Part model, mm, in its own coordinate system. A direction names the side the tool comes from. Coordinates: 2 decimals unless noted, no trailing zeros. Write each loop counter-clockwise with the first axis right and the second up, starting at its lowest first coordinate (ties: lowest second). Pieces come first, ordered by that corner, then holes. Notation, with made-up numbers: M 67,50.25 L 90,50.25 A6 cw 90,58.25 Z; hole C 80,-39 d5. An arc over 180 degrees is marked long. Use a Markdown table: item, result. Add a question column.
Q1. Slice it at B-B on x = -5. Write the cut outline in (y, z).
Q2. Wall check: L1, parallel to X at y = 1, z = -22; L2, parallel to Z at x = 37, y = 2.25; L3, parallel to Y at x = -56.5, z = -41. Give the ranges that are in metal, low to high. Write a range as from..to.
Q3. Pin check, flat tips, straight feed: pin 1 Ø4 at (x, y) = (-13.5, -3.5) entering from +Z; pin 2 Ø5.5 at (x, y) = (-5, -10) entering from +Z; pin 3 Ø7.5 at (y, z) = (0, 23) entering from -X; pin 4 Ø1.8 at (x, z) = (37, -22) entering from +Y. Stop position of each tip, or through.
Q4. Mould opens along Y. For faces 4 (the flat face through (-2, -7, -23)), 5 (the flat face through (-7, -8, -4)), 6 (the flat face through (-38, 5, 23)) say: released by +Y, released by -Y, zero draft, split by the parting line, or undercut.
Q5. Slice it at A-A on y = -0.75. Write the cut outline in (x, z).
Q6. Slice it at C-C on z = -52. Write the cut outline in (x, y).
Q7. Slice it at D-D on x = -21.5. Write the cut outline in (y, z), then the cut area to 4 significant figures.
Q8. Tool access for faces 1 (the flat face through (-55, -10, -35)), 2 (the flat face through (-8, -7, -23)), 3 (the flat face through (-3, -12, 1)): list every direction of +Z, -Z, +X, -X, +Y, -Y with a clear straight run to the whole face (end or side of a thin tool).
Autodesk Inventor part; units mm, degrees
ref_plane "YZ Plane" through (0, 0, 0) normal (1, 0, 0) x (0, 1, 0)
ref_plane "XZ Plane" through (0, 0, 0) normal (0, 1, 0) x (-1, 0, 0)
ref_plane "XY Plane" through (0, 0, 0) normal (0, 0, 1) x (1, 0, 0)
sketch "Sketch1" plane through (0, 0, 0) normal (0, 1, 0) x (-1, 0, 0)
  line L0 (34, 19) -> (-34, 19)
  line L1 (-34, 19) -> (-34, -19)
  line L2 (-34, -19) -> (34, -19)
  line L3 (34, -19) -> (34, 19)
  line L4 (34, 19) -> (-34, -19) construction
  line L5 (-34, 19) -> (34, -19) construction
  line L6 (41, 26) -> (-41, 26)
  line L7 (-41, 26) -> (-41, -26)
  line L8 (-41, -26) -> (41, -26)
  line L9 (41, -26) -> (41, 26)
  line L10 (41, 26) -> (-41, -26) construction
  line L11 (-41, 26) -> (41, -26) construction
  line L12 (-34, -19) -> (-41, -19)
  line L13 (-34, -19) -> (-34, -26)
  line L14 (-34, 19) -> (-41, 19)
  line L15 (-34, 19) -> (-34, 26)
  line L16 (34, -19) -> (34, -26)
  line L17 (34, -19) -> (41, -19)
  line L18 (34, 19) -> (41, 19)
  line L19 (34, 19) -> (34, 26)
  point P0 (0, 0)
  dimension "d0" = 68
  dimension "d1" = 38
  dimension "d2" = 82
  dimension "d3" = 52
extrude "Extrusion1" add sketch "Sketch1" along normal mid plane 10 contours L19 L6 L9 L18 | L14 L7 L6 L15 | L17 L9 L8 L16 | L13 L8 L7 L12
sketch "Sketch2" plane through (0, -5, 0) normal (0, -1, 0) x (1, 0, 0)
  line L0 (-65, -71.5) -> (55, -71.5)
  line L1 (55, -71.5) -> (55, 31)
  line L2 (55, 31) -> (-65, 31)
  line L3 (-65, 31) -> (-65, -71.5)
  line L4 (-34, 26) -> (-41, 26)
  point P0 (0, 0)
  dimension "d6" = 120
  dimension "d7" = 102.5
  dimension "d8" = 5
  dimension "d9" = 55
extrude "Extrusion2" add sketch "Sketch2" along normal blind 10
sketch "Sketch3" plane through (-65, -5, 31) normal (0, 0, 1) x (1, 0, 0)
  circle A0 centre (60, -5) radius 4
  line L0 (120, -10) -> (0, -10)
  line L1 (120, 0) -> (120, -10)
  circle A1 centre (60, -5) radius 2.55
  circle A2 centre (60, -5) radius 3
  line L2 (56, -5) -> (56, -10)
  line L3 (64, -5) -> (64, -10)
  line L4 (56, -10) -> (64, -10)
  point P0 (65, 5)
  point P1 (60, -10)
  dimension "d13" = 8
  dimension "d14" = 5
  dimension "d16" = 5.1
  dimension "d17" = 6
extrude "Extrusion3" cut sketch "Sketch3" against normal blind 30 contours A0 | L3 L0 L2 A0 | A1 | A2
extrude "Extrusion4" cut sketch "Sketch3" against normal blind 60 contours A1
ref_plane "Work Plane2" through (-65, -5, -4) normal (0, 0, 1) x (1, 0, 0)
sketch "Sketch5" plane through (-65, -5, -4) normal (0, 0, 1) x (1, 0, 0)
  circle A0 centre (60, -5) radius 3
  point P0 (65, 5)
extrude "Extrusion5" cut sketch "Sketch5" against normal up to surface (25 mm away)
sketch "Sketch6" plane through (0, -5, 0) normal (0, 1, 0) x (1, 0, 0)
  line L0 (-2, 4) -> (-2, 29)
  line L1 (-2, 29) -> (-8, 29)
  line L2 (-8, 4) -> (-8, 29)
  line L3 (-2, 9) -> (-8, 9)
  point P0 (0, 0)
  dimension "d25" = 20
extrude "Extrusion6" cut sketch "Sketch6" against normal blind 5
fillet "Fillet1" [suppressed]
chamfer "Chamfer1" distance 7.5 angle 45 1 edges at (-5, -5, -29)
sketch "Sketch7" plane through (0, 5, 0) normal (0, 1, 0) x (1, 0, 0)
  circle A0 centre (37, 22) radius 1.6
  circle A1 centre (37, -22) radius 1.6
  circle A2 centre (-37, -22) radius 1.6
  point P0 (0, 0)
  point P1 (-37, 22)
hole "Hole1" at (37, 5, -22) at (37, 5, 22) at (-37, 5, 22) at (-37, 5, -22) direction (0, -1, 0) diameter 2 depth 8 tip angle 118
sketch "Sketch8" plane through (0, -5, 0) normal (0, 1, 0) x (1, 0, 0)
  line L0 (-65, -31) -> (-55, -31)
  line L1 (-55, -31) -> (-55, -8)
  line L2 (-55, -8) -> (-65, -8)
  line L3 (-65, -8) -> (-65, -31)
  line L4 (-65, -31) -> (-65, 71.5)
  line L5 (-65, 71.5) -> (-55, 71.5)
  line L6 (-55, 71.5) -> (-55, 48.5)
  line L7 (-55, 48.5) -> (-65, 48.5)
  line L8 (-65, 48.5) -> (-65, 71.5)
  line L9 (55, -31) -> (-65, -31)
  line L10 (55, -31) -> (45, -31)
  line L11 (45, -31) -> (45, -8)
  line L12 (45, -8) -> (55, -8)
  line L13 (55, -8) -> (55, -31)
  point P0 (0, 0)
  dimension "d39" = 10
  dimension "d40" = 23
  dimension "d41" = 10
  dimension "d42" = 23
  dimension "d43" = 10
  dimension "d44" = 23
sketch "Sketch9" plane through (55, -5, -71.5) normal (0, 0, -1) x (-1, 0, 0)
  line L0 (120, 0) -> (120, -10)
  line L1 (120, -2.5) -> (110, -2.5)
  line L2 (110, -2.5) -> (110, -7.5)
  line L3 (110, -7.5) -> (120, -7.5)
  line L4 (120, -7.5) -> (120, -2.5)
  line L5 (0, 0) -> (0, -10)
  line L6 (0, -2.5) -> (10, -2.5)
  line L7 (10, -2.5) -> (10, -7.5)
  line L8 (10, -7.5) -> (0, -7.5)
  line L9 (0, -7.5) -> (0, -2.5)
  point P0 (55, 5)
  point P1 (110, -5)
  point P2 (120, -5)
  point P3 (10, -5)
  point P4 (0, -5)
  point P5 (0, -7.5)
  dimension "d45" = 5
  dimension "d46" = 10
  dimension "d47" = 10
  dimension "d48" = 5
extrude "Extrusion7" cut sketch "Sketch9" against normal blind 75
delete_face "Delete Face1" [suppressed]
properties part number "PCB_Housing_01_V3"
Recorded:
| question | item | result |
|---|---|---|
| 1 | outline | M -15,-71.5 L -5,-71.5 L -5,-36.5 L -12.5,-29 L -13,-29 L -13,-4 L -12.55,-4 L -12.55,1 L -15,1 Z; M -7.45,-4 L -7,-4 L -7,-9 L -5,-9 L -5,31 L -6,31 L -6,1 L -7.45,1 Z |
| 2 | L1 | -41..-38, -36..-34, 34..36, 38..41 |
| 2 | L2 | -26..-23, -21..-19, 19..21, 23..26 |
| 2 | L3 | -15..-12.5, -7.5..-5 |
| 3 | pin 1 | z = 31 |
| 3 | pin 2 | z = 1 |
| 3 | pin 3 | x = -41 |
| 3 | pin 4 | y = -3.06 |
| 4 | face 4 | zero draft |
| 4 | face 5 | undercut |
| 4 | face 6 | released by +Y |
| 5 | outline | M -41,-26 L -34,-26 L -34,-19 L -41,-19 Z; M -41,19 L -34,19 L -34,26 L -41,26 Z; M 34,-26 L 41,-26 L 41,-19 L 34,-19 Z; M 34,19 L 41,19 L 41,26 L 34,26 Z; hole C -37,-22 d2; hole C -37,22 d2; hole C 37,-22 d2; hole C 37,22 d2 |
| 6 | outline | M -65,-15 L 55,-15 L 55,-12.5 L 45,-12.5 L 45,-7.5 L 55,-7.5 L 55,-5 L -65,-5 L -65,-7.5 L -55,-7.5 L -55,-12.5 L -65,-12.5 Z |
| 7 | outline | M -15,-71.5 L -5,-71.5 L -5,31 L -15,31 Z |
| 7 | area | 1,025 mm² |
| 8 | face 1 | -Z, -X |
| 8 | face 2 | +Y |
| 8 | face 3 | +Z, -Y |
